Design review of the part shown in the three views and the two pictorial views. Dimensions are in mm from the part's minimum x, y and z. Give positions to 0.01 mm unless a question says otherwise; leave off trailing zeros. Order: outer loops, then holes, each group sorted by start corner. A loop starts at its lowest first (then second) coordinate and runs counter-clockwise, first axis right, second up. Notation, with made-up numbers: (6, -14) -> (57, -14) arc R15 cw to (57, -2) -> close; hole circle Ø10 at (77.25, 43). An arc over 180 degrees is marked (long way). Use one line per item in the form item = value.
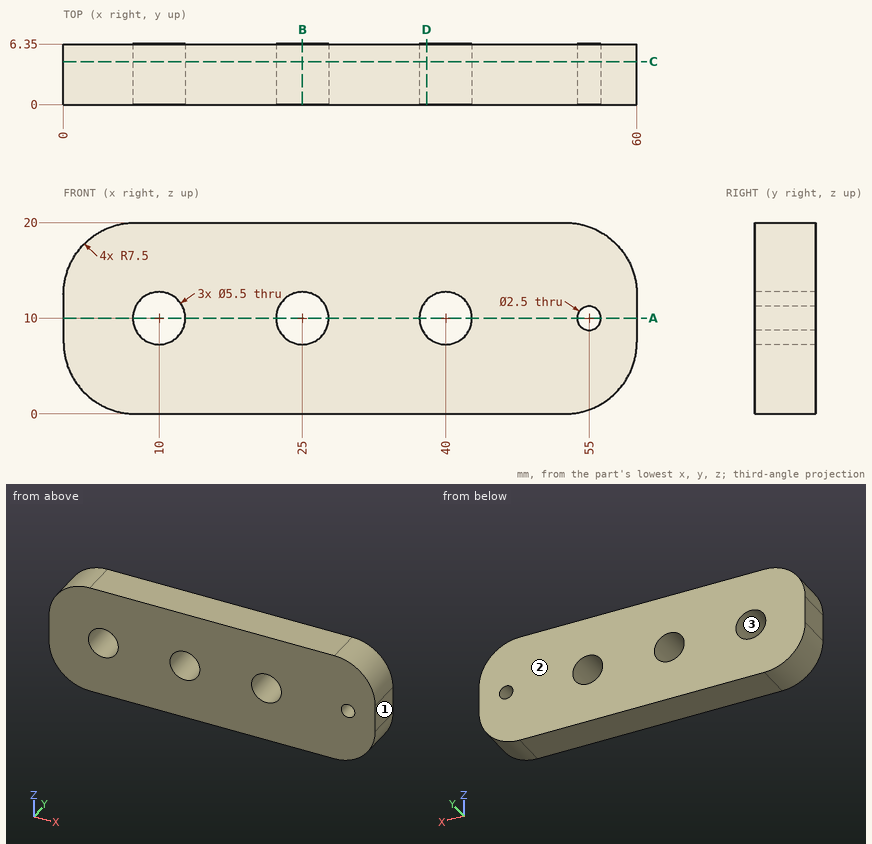
1. Add section A-A on z = 10. Give the boundary of the cut face in (x, y), then the cut area to 3 significant figures.
Values:
outline = (0, 0) -> (7.25, 0) -> (7.25, 6.35) -> (0, 6.35) -> close; (12.75, 0) -> (22.25, 0) -> (22.25, 6.35) -> (12.75, 6.35) -> close; (27.75, 0) -> (37.25, 0) -> (37.25, 6.35) -> (27.75, 6.35) -> close; (42.75, 0) -> (53.75, 0) -> (53.75, 6.35) -> (42.75, 6.35) -> close; (56.25, 0) -> (60, 0) -> (60, 6.35) -> (56.25, 6.35) -> close
area = 260 mm^2
2. For L1, parallel to X at y = 2, z = 10; L2, parallel to X at y = 2, z = 10.5; L3, parallel to Z at x = 26, y = 3.25, list the stretches that pass through material, from the lowest coordinate up.
Values:
L1 = 0 to 7.25, 12.75 to 22.25, 27.75 to 37.25, 42.75 to 53.75, 56.25 to 60
L2 = 0 to 7.3, 12.7 to 22.3, 27.7 to 37.3, 42.7 to 53.85, 56.15 to 60
L3 = 0 to 7.44, 12.56 to 20
3. Add section D-D on x = 38. Give the boundary of the cut face in (y, z).
Values:
outline = (0, 0) -> (6.35, 0) -> (6.35, 8.11) -> (0, 8.11) -> close; (0, 11.89) -> (6.35, 11.89) -> (6.35, 20) -> (0, 20) -> close
4. For pin 1 Ø2 at (x, z) = (55, 10) entering from -Y, flat-tipped, find the tip position at first contact; note if it passes through.
Values:
pin_1 = through
5. Add section C-C on y = 4.5. Give the boundary of the cut face in (x, z).
Values:
outline = (0, 7.5) arc R7.5 ccw to (7.5, 0) -> (52.5, 0) arc R7.5 ccw to (60, 7.5) -> (60, 12.5) arc R7.5 ccw to (52.5, 20) -> (7.5, 20) arc R7.5 ccw to (0, 12.5) -> close; hole circle Ø5.5 at (10, 10); hole circle Ø5.5 at (25, 10); hole circle Ø5.5 at (40, 10); hole circle Ø2.5 at (55, 10)
6. Add section B-B on x = 25. Give the boundary of the cut face in (y, z).
Values:
outline = (0, 0) -> (6.35, 0) -> (6.35, 7.25) -> (0, 7.25) -> close; (0, 12.75) -> (6.35, 12.75) -> (6.35, 20) -> (0, 20) -> close
7. The part is to be moulded in two halves that separate along X. For the marked faces 1, 2 and 3, say which applies: +X half, -X half, draft (parallel to the pull), parting line (faces both ways), or undercut.
Values:
face_1 = +X half
face_2 = draft
face_3 = undercut
